Could you check a few things on this model? Use its own coordinates, in mm. A direction names the side the tool comes from. Round coordinates to 2 decimals unless told otherwise and drop trailing zeros.
Autodesk Inventor part; units mm, degrees
ref_plane "YZ Plane" through (0, 0, 0) normal (1, 0, 0) x (0, 1, 0)
ref_plane "XZ Plane" through (0, 0, 0) normal (0, 1, 0) x (-1, 0, 0)
ref_plane "XY Plane" through (0, 0, 0) normal (0, 0, 1) x (1, 0, 0)
sketch "Szkic1" plane through (0, 0, 0) normal (0, 0, 1) x (1, 0, 0)
  line L0 (-13.9027, 6.9311) -> (286.0973, 6.9311)
  line L1 (286.0973, 6.9311) -> (286.0973, -273.0689)
  line L2 (286.0973, -273.0689) -> (-13.9027, -273.0689)
  line L3 (-13.9027, -273.0689) -> (-13.9027, 6.9311)
  point P0 (0, 0)
  dimension "d0" = 300
  dimension "d1" = 280
extrude "Wyciągnięcie proste1" add sketch "Szkic1" along normal blind 6
sketch "Szkic2" plane through (0, 0, 6) normal (0, 0, 1) x (1, 0, 0)
  line L0 (286.0973, 6.9311) -> (-13.9027, 6.9311)
  line L1 (-13.9027, 6.9311) -> (-13.9027, -273.0689)
  line L2 (-13.9027, -273.0689) -> (286.0973, -273.0689)
  line L3 (286.0973, -273.0689) -> (286.0973, 6.9311)
  point P0 (0, 0)
  point P1 (-2.9027, -39.5689)
  point P2 (275.0973, -39.5689)
  point P3 (-2.9027, -223.0689)
  point P4 (275.0973, -223.0689)
  dimension "d4" = 46.5
  dimension "d5" = 300
  dimension "d6" = 46.5
  dimension "d7" = 11
  dimension "d8" = 11
  dimension "d9" = 50
  dimension "d10" = 50
  dimension "d11" = 11
  dimension "d12" = 11
hole "Otwór1" at (-2.9027, -39.5689, 6) at (275.0973, -39.5689, 6) at (-2.9027, -223.0689, 6) at (275.0973, -223.0689, 6) direction (0, 0, -1) diameter 4 end through all
hole "Otwór2" at (-2.9027, -39.5689, 6) at (275.0973, -39.5689, 6) at (-2.9027, -223.0689, 6) at (275.0973, -223.0689, 6) direction (0, 0, -1) diameter 8 depth 3 tip angle 118
properties part number "CNCM_ALU_6mm_Heatbed"
Item 1: If I drill on line 1 along X through (y, z) = (-41, 1.8), over which ranges is the centre line in solid material (lowest first)?
Results list:
line 1: x = -13.9 to -4.3, -1.5 to 273.7, 276.5 to 286.1
Item 2: We'd pull the mould along X, two halves only. Please class faces 1 (the flat face through (134, -131, 6)), 2 (the cylindrical face through (-4.104, -43.384, 4.479)): released by +X, released by -X, zero draft, split by the parting line, or undercut.
Results list:
face 1: zero draft
face 2: undercut
Item 3: For faces 3 (the cylindrical face through (-5.606, -220.121, 4.479)), 4 (the flat face through (134, -131, 0)), which set-ups out of +Z, -Z, +X, -X, +Y, -Y let a thin tool reach every point of the face, with its end or its side?
Results list:
face 3: +Z
face 4: -Z, +X, -X, +Y, -Y
Item 4: Will this pin go through, and if not, where does the flat tip stop? pin 1 (5 mm diameter, centred on x = -2.9, y = -39.57, fed in from +Z).
Results list:
pin 1: stops at z = 2.1
